Geometry: final body of the model. Coordinates: model frame, mm. A direction names the side the tool comes from. Coordinates: 2 decimals unless noted, no trailing zeros. Order: outer loops, then holes, each group sorted by start corner. A loop starts at its lowest first (then second) coordinate and runs counter-clockwise, first axis right, second up. Notation, with made-up numbers: (73.5, 49) -> (89.5, 49) arc R13 cw to (89.5, 63) -> close; hole circle Ø5 at (28.25, 22). An arc over 180 degrees is marked (long way). Use one line per item in the form item = value.
```python
from build123d import *

# Parameters (mm, degrees)
BOSS_EXTRUDE1_DEPTH = 7
SKETCH2_W           = 29.216076644
SKETCH2_H           = 30
CUT_EXTRUDE1_DEPTH  = 4.46
FILLET1_R           = 2.54
FILLET2_R           = 1.27
CUT_EXTRUDE2_REACH  = 9
SKETCH3_R           = 2.54
SKETCH3_W           = 5.08
SKETCH3_H           = 12.7
CHAMFER1_SIZE       = 1.27
SKETCH4_R           = 1.27
CUT_EXTRUDE3_DEPTH  = 31


with BuildPart() as part:
    # Sketch1 → Boss-Extrude1 (new body)
    with BuildSketch(Plane(origin=(0, 0, 0), x_dir=(1, 0, 0), z_dir=(0, 1, 0))):
        with BuildLine():
            Line((0, 0), (21.000000028, 0))
            ThreePointArc((21.000000028, 0), (36.000000028, 15), (21.000000028, 30))
            Line((21.000000028, 30), (0, 30))
            Line((0, 30), (0, 0))
        make_face()
    extrude(amount=BOSS_EXTRUDE1_DEPTH)

    # Sketch2 → Cut-Extrude1 (cut)
    with BuildSketch(Plane.XZ):
        with Locations((21.608038322, -15)):
            Rectangle(SKETCH2_W, SKETCH2_H)
    extrude(amount=-CUT_EXTRUDE1_DEPTH, mode=Mode.SUBTRACT)

    # Fillet1
    fillet1_edges = [part.edges().sort_by_distance(p)[0] for p in [
        (7, 0, -15),
    ]]
    fillet(fillet1_edges, radius=FILLET1_R)

    # Fillet2
    fillet2_edges = [part.edges().sort_by_distance(p)[0] for p in [
        (0, 7, -15),
        (0, 0, -15),
    ]]
    fillet(fillet2_edges, radius=FILLET2_R)

    # Sketch3 → Cut-Extrude2 (cut, up to next)
    with BuildSketch(Plane(origin=(0, 7, 0), x_dir=(1, 0, 0), z_dir=(0, 1, 0)), mode=Mode.PRIVATE) as cut_extrude2_sk1:
        with Locations((28.34999918, 15)):
            Circle(SKETCH3_R)
    cut_extrude2_tool1 = extrude(cut_extrude2_sk1.sketch, amount=-CUT_EXTRUDE2_REACH, mode=Mode.PRIVATE) & part.part
    add(cut_extrude2_tool1.solids().sort_by_distance((28.349999, 7, -15))[0], mode=Mode.SUBTRACT)
    # Sketch3 → Cut-Extrude2 (cut, up to next)
    with BuildSketch(Plane(origin=(0, 7, 0), x_dir=(1, 0, 0), z_dir=(0, 1, 0)), mode=Mode.PRIVATE) as cut_extrude2_sk2:
        with Locations((19.3499994, 23.99999978)):
            Circle(SKETCH3_R)
    cut_extrude2_tool2 = extrude(cut_extrude2_sk2.sketch, amount=-CUT_EXTRUDE2_REACH, mode=Mode.PRIVATE) & part.part
    add(cut_extrude2_tool2.solids().sort_by_distance((19.349999, 7, -24))[0], mode=Mode.SUBTRACT)
    # Sketch3 → Cut-Extrude2 (cut, up to next)
    with BuildSketch(Plane(origin=(0, 7, 0), x_dir=(1, 0, 0), z_dir=(0, 1, 0)), mode=Mode.PRIVATE) as cut_extrude2_sk3:
        with Locations((19.3499994, 6.00000022)):
            Circle(SKETCH3_R)
    cut_extrude2_tool3 = extrude(cut_extrude2_sk3.sketch, amount=-CUT_EXTRUDE2_REACH, mode=Mode.PRIVATE) & part.part
    add(cut_extrude2_tool3.solids().sort_by_distance((19.349999, 7, -6))[0], mode=Mode.SUBTRACT)
    # Sketch3 → Cut-Extrude2 (cut, up to next)
    with BuildSketch(Plane(origin=(0, 7, 0), x_dir=(1, 0, 0), z_dir=(0, 1, 0)), mode=Mode.PRIVATE) as cut_extrude2_sk4:
        with Locations((2.54, 15)):
            Rectangle(SKETCH3_W, SKETCH3_H)
    cut_extrude2_tool4 = extrude(cut_extrude2_sk4.sketch, amount=-CUT_EXTRUDE2_REACH, mode=Mode.PRIVATE) & part.part
    add(cut_extrude2_tool4.solids().sort_by_distance((2.54, 7, -15))[0], mode=Mode.SUBTRACT)

    # Chamfer1
    chamfer1_edges = [part.edges().sort_by_distance(p)[0] for p in [
        (25.80999918, 7, -15),
        (16.8099994, 7, -23.99999978),
        (16.8099994, 7, -6.00000022),
    ]]
    chamfer(chamfer1_edges, length=CHAMFER1_SIZE)

    # Sketch4 → Cut-Extrude3 (cut, through all)
    with BuildSketch(Plane.XY):
        with Locations((2.54, 4.46)):
            Circle(SKETCH4_R)
    extrude(amount=-CUT_EXTRUDE3_DEPTH, mode=Mode.SUBTRACT)


solid = part.part
```
1) Section B-B, the plane z = -15. Output: boundary loops of the cut face in (x, y).
Results found:
outline = (5.08, 0.08) arc R2.54 ccw to (7, 2.54) -> (7, 4.46) -> (25.81, 4.46) -> (25.81, 5.73) -> (24.54, 7) -> (5.08, 7) -> close; (30.89, 4.46) -> (36, 4.46) -> (36, 7) -> (32.16, 7) -> (30.89, 5.73) -> close
2) Contact query for flat-ended pins moving along their axis: P1, Ø6, axis at x = 32, z = -18.5, coming from the -Y side; P2, Ø4, axis at x = 28.35, z = -15, coming from the -Y side; P3, Ø8, axis at x = 10, z = -8, coming from the -Y side. Output: stop coordinate, or through.
Results found:
P1 = 4.46
P2 = through
P3 = 0.52
3) Section A-A, the plane z = -24. Output: boundary loops of the cut face in (x, y), and give its area (3 significant figures).
Results found:
outline = (0, 1.27) arc R1.27 ccw to (1.27, 0) -> (4.46, 0) arc R2.54 ccw to (7, 2.54) -> (7, 4.46) -> (16.81, 4.46) -> (16.81, 5.73) -> (15.54, 7) -> (1.27, 7) arc R1.27 ccw to (0, 5.73) -> close; (21.89, 4.46) -> (33, 4.46) -> (33, 7) -> (23.16, 7) -> (21.89, 5.73) -> close; hole circle Ø2.54 at (2.54, 4.46)
area = 93.4 mm2
4) Access query for faces 1 (the flat face through (3, 3, -21.35)), 2 (the flat face through (0, 3, -26)), 3 (the flat face through (7, 3, -15)). Directions: +Z, -Z, +X, -X, +Y, -Y. A direction counts if a zero-diameter tool reaches every point of the face in a straight line with its end or side. Return the directions, or none.
Results found:
face_1 = -X, +Y, -Y
face_2 = +Z, -Z, -X, +Y, -Y
face_3 = +Z, -Z, +X, -Y
5) Pull-direction query (Z, two-part tool) for faces 4 (the cylindrical face through (26.3, 5.1, -13.5)), 5 (the flat face through (8, 5, -30)), 6 (the flat face through (0, 3, -4)); classes: released by +Z, released by -Z, zero draft, split by the parting line, or undercut.
Results found:
face_4 = undercut
face_5 = released by -Z
face_6 = zero draft
6) Section D-D, the plane y = 2. Output: boundary loops of the cut face in (x, z).
Results found:
outline = (0, -30) -> (6.94, -30) -> (6.94, 0) -> (0, 0) -> (0, -8.65) -> (5.08, -8.65) -> (5.08, -21.35) -> (0, -21.35) -> close
7) Section C-C, the plane x = 19.35. Give the number of separate pieces and of enclosed holes in the cut face, and give its area (3 significant figures).
Results found:
separate_pieces = 3
enclosed_holes = 0
area = 47.2 mm2
8) Material intervals for probe 1 along Z at (x, y) = (19.35, 4.85); probe 2 along X at (y, z) = (5.3, -15); probe 3 along Y at (x, z) = (2.54, -26.75), sorted ascending. Write a range as from..to.
Results found:
probe_1 = -30..-26.54, -21.46..-8.54, -3.46..0
probe_2 = 5.08..25.81, 30.89..36
probe_3 = 0..3.19, 5.73..7
